```python
from build123d import *

# Parameters (mm, degrees)
F0_R     = 8
F1_DEPTH = 450
F2_R     = 4
F3_DEPTH = 60
F4_R     = 4
F5_DEPTH = 60


with BuildPart() as f1:
    # F0 (on Front) → F1 (new body, symmetric)
    with BuildSketch(Plane.XZ):
        Circle(F0_R)
    extrude(amount=F1_DEPTH, both=True)

    # F2 (on face) → F3 (cut)
    with BuildSketch(Plane.XZ.offset(450)):
        Circle(F2_R)
    extrude(amount=-F3_DEPTH, mode=Mode.SUBTRACT)

    # F4 (on face) → F5 (cut)
    with BuildSketch(Plane(origin=(0, 450, 0), x_dir=(-1, 0, 0), z_dir=(0, 1, 0))):
        Circle(F4_R)
    extrude(amount=-F5_DEPTH, mode=Mode.SUBTRACT)


solid = f1.part
```
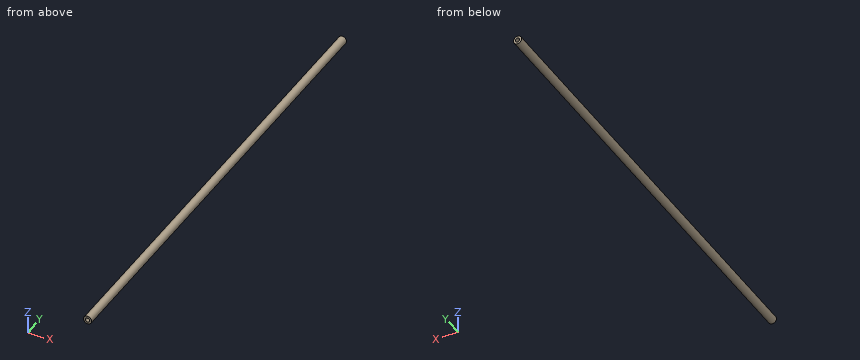
Verification items for the finished model (mm, model axes). Round coordinates to 2 decimals unless told otherwise and drop trailing zeros. Order: outer loops, then holes, each group sorted by start corner. A loop starts at its lowest first (then second) coordinate and runs counter-clockwise, first axis right, second up.
1) Cross-section at B-B, the plane x = 0. Record the cut outline in (y, z).
Geometry says:
outline: (-450, -8) - (450, -8) - (450, -4) - (390, -4) - (390, 4) - (450, 4) - (450, 8) - (-450, 8) - (-450, 4) - (-390, 4) - (-390, -4) - (-450, -4) - close
2) Cross-section at C-C, the plane y = 253. Record the cut outline in (x, z), plus the area to 3 significant figures.
Geometry says:
outline: circle Ø16 at (0, 0)
area: 201 mm2
3) Material ranges on line 1 (Z direction, x = 0, y = -427); line 2 (Y direction, x = -0.25, z = -3.5); line 3 (X direction, y = 228, z = -0.25), recorded low to high.
Geometry says:
line 1: z = -8 to -4, 4 to 8
line 2: y = -390 to 390
line 3: x = -8 to 8
4) Cross-section at A-A, the plane z = 0. Record the cut outline in (x, y), plus the area to 3 significant figures.
Geometry says:
outline: (-8, -450) - (-4, -450) - (-4, -390) - (4, -390) - (4, -450) - (8, -450) - (8, 450) - (4, 450) - (4, 390) - (-4, 390) - (-4, 450) - (-8, 450) - close
area: 13,400 mm2
5) Depth check by flat-ended pin: pin 1 (2.5 mm diameter, centred on x = -1.5, z = 2, fed in from +Y); pin 2 (1.5 mm diameter, centred on x = -4.5, y = 225.5, fed in from +Z); pin 3 (1 mm diameter, centred on y = -105.5, z = 2.5, fed in from +X). Enter the tip coordinate at first touch or a pass-through.
Geometry says:
pin 1: stops at y = 390
pin 2: stops at z = 7.07
pin 3: stops at x = 7.75
